Verification items for the finished model (mm, model axes). A direction names the side the tool comes from. Round coordinates to 2 decimals unless told otherwise and drop trailing zeros. Order: outer loops, then holes, each group sorted by start corner. A loop starts at its lowest first (then second) coordinate and runs counter-clockwise, first axis right, second up. Notation, with made-up numbers: (37, -30.75) -> (85, -30.75) arc R17 ccw to (85, -13.75) -> close; hole circle Ø6 at (68.25, -22). An arc over 180 degrees is marked (long way). Put each result on its own line as item: value.
from build123d import *

# Parameters (mm, degrees)
SKETCH1_W           = 100
SKETCH1_H           = 200
BOSS_EXTRUDE1_DEPTH = 10
SKETCH3_W           = 50
SKETCH3_H           = 40
BOSS_EXTRUDE2_DEPTH = 25


with BuildPart() as part:
    # Sketch1 → Boss-Extrude1 (new body)
    with BuildSketch(Plane(origin=(0, 0, 0), x_dir=(1, 0, 0), z_dir=(0, 1, 0))):
        with Locations((50, 100)):
            Rectangle(SKETCH1_W, SKETCH1_H)
    extrude(amount=BOSS_EXTRUDE1_DEPTH)

    # Sketch3 → Boss-Extrude2 (add)
    with BuildSketch(Plane(origin=(0, 10, 0), x_dir=(1, 0, 0), z_dir=(0, 1, 0))):
        with Locations((25, 20)):
            Rectangle(SKETCH3_W, SKETCH3_H)
    extrude(amount=BOSS_EXTRUDE2_DEPTH)

    # Sketch9 → Ø25.0 (25) Diameter Hole2 (revolve, cut)
    with BuildSketch(Plane(origin=(35, 10, -170), x_dir=(0, 0, 1), z_dir=(1, 0, 0))):
        Polygon((0, 0), (0, 10), (12.5, 10), (12.5, 0.025), (12.525, 0), align=None)
    revolve(axis=Axis((35, 16.35, -170), (0, -1, 0)), mode=Mode.SUBTRACT)


solid = part.part
Item 1: Section check B-B on x = 35. Record the boundary of the cut face in (y, z) (3 decimals), then the cut area to 3 significant figures.
Check sheet entries:
outline: (0, -200) -> (10, -200) -> (10, -182.525) -> (9.975, -182.5) -> (0, -182.5) -> close; (0, -157.5) -> (9.975, -157.5) -> (10, -157.475) -> (10, -40) -> (35, -40) -> (35, 0) -> (0, 0) -> close
area: 2,750 mm^2
Item 2: Section check C-C on y = 7. Record the boundary of the cut face in (x, z), then the cut area to 3 significant figures.
Check sheet entries:
outline: (0, -200) -> (100, -200) -> (100, 0) -> (0, 0) -> close; hole circle Ø25 at (35, -170)
area: 19,500 mm^2
Item 3: Section check A-A on z = -170. Record the boundary of the cut face in (x, y) (3 decimals), then the cut area to 3 significant figures.
Check sheet entries:
outline: (0, 0) -> (22.5, 0) -> (22.5, 9.975) -> (22.475, 10) -> (0, 10) -> close; (47.5, 0) -> (100, 0) -> (100, 10) -> (47.525, 10) -> (47.5, 9.975) -> close
area: 750 mm^2
Item 4: Section check D-D on z = -21.5. Record the boundary of the cut face in (x, y).
Check sheet entries:
outline: (0, 0) -> (100, 0) -> (100, 10) -> (50, 10) -> (50, 35) -> (0, 35) -> close
Item 5: Tool access check on faces 1 (the flat face through (25, 22, -40)), 2 (the flat face through (0, 9, -76)), 3 (the flat face through (50, 22, -20)). Record the directions out of +Z, -Z, +X, -X, +Y, -Y that give a thin tool (end or side, any length) a straight path to the whole face; none if there is none.
Check sheet entries:
face 1: -Z, +X, -X, +Y
face 2: +Z, -Z, -X, +Y, -Y
face 3: +Z, -Z, +X, +Y
Item 6: Gauge pin test, flat ends, axial feed: pin 1 Ø12.5 at (x, y) = (30.5, 18) entering from -Z; pin 2 Ø5 at (x, z) = (70, -177) entering from +Y. Record the tip position at first contact, or that the pin passes through.
Check sheet entries:
pin 1: stops at z = -40
pin 2: stops at y = 10
Item 7: Release check for a two-part mould opening along Z. For faces 4 (the flat face through (49, 0, -101)), 5 (the cylindrical face through (31.245, 5.057, -158.077)), 6 (the flat face through (38, 13, 0)) record: +Z half, -Z half, draft (parallel to the pull), parting line (faces both ways), or undercut.
Check sheet entries:
face 4: draft
face 5: undercut
face 6: +Z half
Item 8: Material ranges on L1, parallel to Z at x = 35, y = 7; L2, parallel to X at y = 5, z = -170; L3, parallel to Z at x = 5.5, y = 15, recorded low to high. Write a range as [from, to].
Check sheet entries:
L1: z = [-200, -182.5], [-157.5, 0]
L2: x = [0, 22.5], [47.5, 100]
L3: z = [-40, 0]
